Autodesk Fusion 360 part; units mm, degrees
sketch "Sketch1" plane through (0, 0, 0) normal (0, 0, 1) x (1, 0, 0) in component "Component'"
  line L0 (-12.5, 21.5) -> (12.5, 21.5)
  line L1 (12.5, 21.5) -> (12.5, 19.5)
  line L2 (12.5, 19.5) -> (-12.5, 19.5)
  line L3 (-12.5, 19.5) -> (-12.5, 21.5)
  line L4 (-12.5, -19.5) -> (12.5, -19.5)
  line L5 (12.5, -19.5) -> (12.5, -21.5)
  line L6 (12.5, -21.5) -> (-12.5, -21.5)
  line L7 (-12.5, -21.5) -> (-12.5, -19.5)
  line L8 (0, -19.5) -> (0, 19.5) construction
  line L9 (-4.5, 9) -> (-1.5, 9)
  line L10 (-1.5, 9) -> (-1.5, 6)
  line L11 (-1.5, 6) -> (-4.5, 6)
  line L12 (-4.5, 6) -> (-4.5, 9)
  line L13 (-1.5, 16.5) -> (-1.5, 13.5)
  line L14 (-1.5, 13.5) -> (-4.5, 13.5)
  line L15 (-4.5, 13.5) -> (-4.5, 16.5)
  line L16 (-4.5, 16.5) -> (-1.5, 16.5)
  line L17 (-4.5, -16.5) -> (-4.5, -13.5)
  line L18 (-1.5, -6) -> (-1.5, -9)
  line L19 (-4.5, -6) -> (-1.5, -6)
  line L20 (-4.5, -13.5) -> (-1.5, -13.5)
  line L21 (-4.5, -9) -> (-4.5, -6)
  line L22 (-1.5, -16.5) -> (-4.5, -16.5)
  line L23 (-1.5, -9) -> (-4.5, -9)
  line L24 (-1.5, -13.5) -> (-1.5, -16.5)
  line L25 (-20, 0) -> (15, 0) construction
  line L26 (4.5, 9) -> (4.5, 6)
  line L27 (4.5, 16.5) -> (4.5, 13.5)
  line L28 (1.5, 13.5) -> (1.5, 16.5)
  line L29 (4.5, -16.5) -> (1.5, -16.5)
  line L30 (4.5, -13.5) -> (4.5, -16.5)
  line L31 (1.5, -6) -> (4.5, -6)
  line L32 (4.5, -6) -> (4.5, -9)
  line L33 (1.5, -9) -> (1.5, -6)
  line L34 (1.5, -16.5) -> (1.5, -13.5)
  line L35 (1.5, 6) -> (1.5, 9)
  line L36 (1.5, 9) -> (4.5, 9)
  line L37 (4.5, 6) -> (1.5, 6)
  line L38 (4.5, -9) -> (1.5, -9)
  line L39 (1.5, 16.5) -> (4.5, 16.5)
  line L40 (1.5, -13.5) -> (4.5, -13.5)
  line L41 (4.5, 13.5) -> (1.5, 13.5)
  line L42 (4.5, 19.5) -> (4.5, -19.5)
  line L43 (-4.5, 19.5) -> (-4.5, -19.5)
  line L44 (12.5, 19.5) -> (4.5, 11.5)
  line L45 (12.5, 19.5) -> (24.453, 19.5) construction
  line L46 (-12.5, 19.5) -> (-4.5, 11.5)
  line L47 (-12.5, -19.5) -> (-4.5, -11.5)
  line L48 (12.5, -19.5) -> (4.5, -11.5)
  dimension "d1" = 39
  dimension "d2" = 25
  dimension "d3" = 2
  dimension "d6" = 3
  dimension "d7" = 3
  dimension "d8" = 1.5
  dimension "d9" = 7.5
  dimension "d10" = 3
  dimension "d11" = 3
  dimension "d12" = 7.5
  dimension "d13" = 12
  dimension "d14" = 3
  dimension "d15" = 3
  dimension "d16" = 7.5
  dimension "d17" = 3
  dimension "d18" = 3
  dimension "d19" = 7.5
  dimension "d20" = 12
  dimension "d21" = 135
extrude "Extrude1" add sketch "Sketch1" along normal blind 2 contours L2 L15 L43 L46 | L2 L27 L42 L44 | L2 L4 L9 L10 L11 L13 L14 L16 L18 L19 L20 L22 L23 L24 L28 L29 L31 L33 L34 L35 L36 L37 L38 L39 L40 L41 L42 L43 | L13 L14 L15 L16 L43 | L9 L10 L11 L12 L43 | L27 L28 L39 L41 L42 | L26 L35 L36 L37 L42 | L18 L19 L21 L23 L43 | L31 L32 L33 L38 L42 | L4 L17 L43 L47 | L4 L30 L42 L48 | L17 L20 L22 L24 L43 | L29 L30 L34 L40 L42 in component "Component'"
extrude "Extrude2" add sketch "Sketch1" along normal blind 5 contours L0 L1 L2 L3 | L4 L5 L6 L7 in component "Component'"
extrude "Extrude3" add sketch "Sketch1" against normal blind 5 contours L13 L14 L15 L16 L43 | L9 L10 L11 L12 L43 | L27 L28 L39 L41 L42 | L26 L35 L36 L37 L42 | L18 L19 L21 L23 L43 | L31 L32 L33 L38 L42 | L17 L20 L22 L24 L43 | L29 L30 L34 L40 L42 in component "Component'"
component "Component'" placed x (1, 0, 0) y (0, 1, 0) z (0, 0, 1) at (0, 0, 0)
Geometry check sheet. Reference: the model listing, model coordinates, mm. A direction names the side the tool comes from. Give positions to 0.01 mm unless a question says otherwise; leave off trailing zeros. Loops run counter-clockwise (first coordinate to the right, second up) from the corner with the lowest first, then second, coordinate; pieces in that order, holes last. Notation, with made-up numbers: M 20.5,-27 L 74.5,-27 A21 cw 74.5,-12 Z; hole C 3.25,-36 d4. An arc over 180 degrees is marked long. Answer as a JSON object with one key per item and string values. Group by question number.
Item 1: Access from +Z, -Z, +X, -X, +Y, -Y to the whole of each face (thin tool, end or side, straight path). Record for faces 4 (the flat face through (9, -16, 1)), 5 (the flat face through (-4.5, 0, 1)), 6 (the flat face through (-4.5, -15, -2)), 7 (the flat face through (-3, -6, -2)).
Item 2: Gauge pin test, flat ends, axial feed: pin 1 (1.5 mm diameter, centred on y = -14.5, z = -1.5, fed in from +X); pin 2 (0.9 mm diameter, centred on y = -14.5, z = -3.5, fed in from -X); pin 3 (7.5 mm diameter, centred on x = 5, y = 9, fed in from +Z). Record the tip position at first contact, or that the pin passes through.
Item 3: Sectioned sample at B-B on z = 2.75. Record the boundary of the cut face in (x, y).
Item 4: Sectioned sample at A-A on x = -5.5. Record the boundary of the cut face in (y, z), plus the area to 3 significant figures.
Item 5: Mould release check, pull along Y, two halves, no side actions. Record for faces 1 (the flat face through (-3, 9, -2)), 2 (the flat face through (0, 21, 5)), 3 (the flat face through (3, -16.5, -2)): pulls with the +Y half, pulls with the -Y half, needs draft (parallel to the pull), parting line crosses it, or undercut.
Item 6: Material ranges on L1, parallel to Y at x = 3.25, z = -2.5; L2, parallel to Y at x = 4.25, z = 4; L3, parallel to X at y = 6.5, z = -3, recorded low to high.
Item 7: Sectioned sample at D-D on x = 8.75. Record the boundary of the cut face in (y, z), plus the area to 3 significant figures.
Item 8: Sectioned sample at C-C on z = -1.5. Give the number of separate pieces and of enclosed holes in the cut face, plus the area to 3 significant figures.
Findings below:
{
 "1": {"face 4": "+Z, -Z, +X", "face 5": "+Z, -Z, -X", "face 6": "-Z, -X, +Y, -Y", "face 7": "-Z, +X, -X"},
 "2": {"pin 1": "x = 4.5", "pin 2": "x = -4.5", "pin 3": "z = 2"},
 "3": {"outline": "M -12.5,-21.5 L 12.5,-21.5 L 12.5,-19.5 L -12.5,-19.5 Z; M -12.5,19.5 L 12.5,19.5 L 12.5,21.5 L -12.5,21.5 Z"},
 "4": {"outline": "M -21.5,0 L -12.5,0 L -12.5,2 L -19.5,2 L -19.5,5 L -21.5,5 Z; M 12.5,0 L 21.5,0 L 21.5,5 L 19.5,5 L 19.5,2 L 12.5,2 Z", "area": "48.0 mm2"},
 "5": {"face 1": "undercut", "face 2": "needs draft", "face 3": "pulls with the -Y half"},
 "6": {"L1": "-16.5 to -13.5, -9 to -6, 6 to 9, 13.5 to 16.5", "L2": "-21.5 to -19.5, 19.5 to 21.5", "L3": "-4.5 to -1.5, 1.5 to 4.5"},
 "7": {"outline": "M -21.5,0 L -15.75,0 L -15.75,2 L -19.5,2 L -19.5,5 L -21.5,5 Z; M 15.75,0 L 21.5,0 L 21.5,5 L 19.5,5 L 19.5,2 L 15.75,2 Z", "area": "35.0 mm2"},
 "8": {"separate pieces": "8", "enclosed holes": "0", "area": "72.0 mm2"}
}
